```python
from build123d import *

# Parameters (mm, degrees)
SKETCH2_R          = 0.425
CUT_EXTRUDE2_DEPTH = 10


with BuildPart() as part:
    # Sweep4: sweep along a path in Sketch4
    with BuildLine(Plane(origin=(0, 0, 0), x_dir=(1, 0, 0), z_dir=(0, 1, 0))) as sweep4_path:
        Line((67.536722789, 33.517901337), (63.696993057, 30.160880485))
        ThreePointArc((63.696993057, 30.160880485), (62.67844941, 29.718218887), (61.591563938, 29.94638641))
        Line((61.591563938, 29.94638641), (58.647554869, 31.613971966))
        ThreePointArc((58.647554869, 31.613971966), (57.417647247, 32.11454889), (56.100779486, 32.285163408))
    # Sketch2 → Sweep4 (sweep)
    with BuildSketch(Plane(origin=(50.527312063, 4.259e-06, -50.527312063), x_dir=(0.707106781, 0, 0.707106781), z_dir=(0.707106781, 6e-08, -0.707106781))):
        with Locations((24.054939337, 4.259e-06)):
            Circle(SKETCH2_R)
    sweep(path=sweep4_path.line)

    # Sketch6 → Revolve1 (revolve)
    with BuildSketch(Plane(origin=(0, 0, 0), x_dir=(1, 0, 0), z_dir=(0, 1, 0))):
        Polygon((56.100779486, 32.285163408), (31.850231497, 32.285163408), (11.591647887, 32.285163408), (-52.408352113, 32.285163408), (-72.666935722, 32.285163408), (-96.917483711, 32.285163408), (-96.917483711, 31.785163408), (-72.666935722, 31.085163408), (-72.666935722, 30.485163408), (-52.408352113, 30.285163408), (-52.408352113, 29.785163408), (11.591647887, 29.785163408), (11.591647887, 30.285163408), (31.850231497, 30.485163408), (31.850231497, 31.085163408), (56.100779486, 31.785163408), align=None)
    revolve(axis=Axis((11.591647887, 0, -32.285163408), (-1, 0, 0)))

    # Sketch7 → Cut-Extrude2 (cut)
    with BuildSketch(Plane(origin=(12.979011819, 0, 14.845274956), x_dir=(-0.752843126, 0, 0.65819999), z_dir=(-0.65819999, 0, -0.752843126))):
        with BuildLine():
            Line((-70.90689286, -0.258658753), (-70.424884302, -0.480296071))
            Line((-70.424884302, -0.480296071), (-73.177134487, -0.809094289))
            Line((-73.177134487, -0.809094289), (-73.643040117, 0.425))
            Line((-73.643040117, 0.425), (-71.097248445, 0.425))
            ThreePointArc((-71.097248445, 0.425), (-71.956470511, 0.264804948), (-72.71646768, -0.166853846))
            Line((-72.71646768, -0.166853846), (-72.763912994, -0.258658753))
            ThreePointArc((-72.763912994, -0.258658753), (-71.835402927, -0.055413386), (-70.90689286, -0.258658753))
        make_face()
    extrude(amount=CUT_EXTRUDE2_DEPTH, mode=Mode.SUBTRACT)


solid = part.part
```
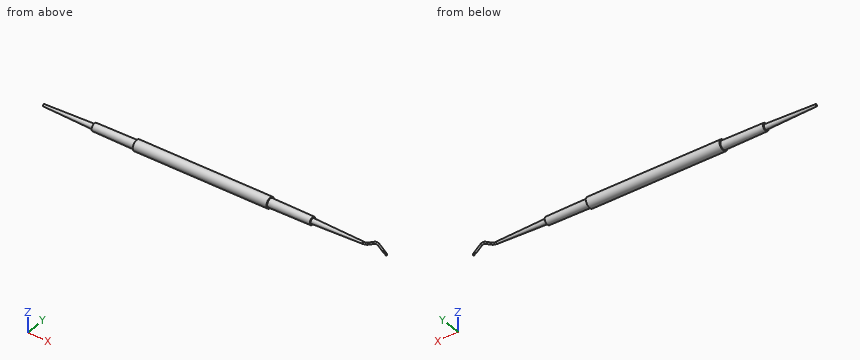
For this review, take the finished solid that the model builds, in its own axes (mm). Coordinates: 2 decimals unless noted, no trailing zeros. Write each loop counter-clockwise with the first axis right and the second up, starting at its lowest first coordinate (ties: lowest second). Pieces come first, ordered by that corner, then holes.
(1) Add section A-A on x = 2. Give the boundary of the cut face in (y, z).
(2) Wall thickness on probe 1 along X at (y, z) = (-0.55, -30.9); probe 2 along Y at (x, z) = (-27, -32.1); probe 3 along Z at (x, y) = (-42.5, 0.1): over which ranges is each line inside the solid? List them lowest first.
(3) For pin 1 Ø1.5 at (x, z) = (-45.5, -34) entering from -Y; pin 2 Ø0.8 at (y, z) = (0, -32) entering from +X; pin 3 Ø1 at (x, z) = (12, -33) entering from -Y; pin 4 Ø1.5 at (y, z) = (1, -32.5) entering from -X, all flat-tipped, find the tip position at first contact; note any pin that passes through.
(4) Add section B-B on x = 18.5. Give the boundary of the cut face in (y, z), then the cut area to 3 significant figures.
Answer sheet:
1. outline: circle Ø5 at (0, -32.29)
2. probe 1: x = -72.67 to 31.85
2. probe 2: y = -2.49 to 2.49
2. probe 3: z = -34.78 to -29.79
3. pin 1: stops at y = -2.31
3. pin 2: stops at x = 66.9
3. pin 3: stops at y = -2.46
3. pin 4: stops at x = -96.92
4. outline: circle Ø3.86 at (0, -32.29)
4. area: 11.7 mm2
